Design review of the part built by this model. Coordinates are the model's own, in mm. A direction names the side the tool comes from. Coordinates: 2 decimals unless noted, no trailing zeros. Loops run counter-clockwise (first coordinate to the right, second up) from the corner with the lowest first, then second, coordinate; pieces in that order, holes last. Notation, with made-up numbers: (8, 70.5) -> (21, 70.5) arc R18 ccw to (21, 80.5) -> close; hole circle Ø10 at (31.25, 52). An arc over 180 degrees is marked (long way). Answer in a Markdown table with one row per item.
```python
from build123d import *

# Parameters (mm, degrees)
CHAMFER_1_SIZE      = 0.2
CHAMFER_2_SIZE      = 0.2
CUT_EXTRUDE_1_DEPTH = 2.4
EXTRUDE_2_REACH     = 21
SKETCH_4_R          = 1.832050808


with BuildPart() as part:
    # Sketch S → Revolve D (revolve)
    with BuildSketch(Plane(origin=(0, 0, 0), x_dir=(-1, 0, 0), z_dir=(0, 1, 0))):
        Polygon((0, 0), (2.75, 0), (2.75, -3), (1.5, -3), (1.5, -19), (0, -19), align=None)
    revolve(axis=Axis((0, 0, 20), (0, 0, -1)))

    # Chamfer 1
    chamfer_1_edges = [part.edges().sort_by_distance(p)[0] for p in [
        (2.75, 0, 0),
    ]]
    chamfer(chamfer_1_edges, length=CHAMFER_1_SIZE)

    # Chamfer 2
    chamfer_2_edges = [part.edges().sort_by_distance(p)[0] for p in [
        (1.5, 0, -19),
    ]]
    chamfer(chamfer_2_edges, length=CHAMFER_2_SIZE)

    # Sketch 2 → Cut-Extrude 1 (cut)
    with BuildSketch(Plane(origin=(0, 0, 0), x_dir=(0, 1, 0), z_dir=(0, 0, 1))):
        Polygon((0, 1.732050808), (1.5, 0.866025404), (1.5, -0.866025404), (0, -1.732050808), (-1.5, -0.866025404), (-1.5, 0.866025404), align=None)
    extrude(amount=-CUT_EXTRUDE_1_DEPTH, mode=Mode.SUBTRACT)

    # Sketch 3 → Cut-Revolve 1 (revolve, cut)
    with BuildSketch(Plane(origin=(0, 0, 0), x_dir=(1, 0, 0), z_dir=(0, 1, 0))):
        Polygon((-1.832050808, 0), (0, 0), (0, 3.4), (-1.832050808, 2.342264973), align=None)
    revolve(axis=Axis((0, 0, -30.07825812), (0, 0, 1)), mode=Mode.SUBTRACT)

    # Sketch 4 → Extrude 2 (add, up to next)
    with BuildSketch(Plane.XY, mode=Mode.PRIVATE) as extrude_2_sk1:
        Circle(SKETCH_4_R)
        Polygon((-1.732050808, 0), (-0.866025404, 1.5), (0.866025404, 1.5), (1.732050808, 0), (0.866025404, -1.5), (-0.866025404, -1.5), align=None, mode=Mode.SUBTRACT)
    extrude_2_tool1 = extrude(extrude_2_sk1.sketch, amount=-EXTRUDE_2_REACH, mode=Mode.PRIVATE) - part.part
    add(extrude_2_tool1.solids().sort_by_distance((-1.780233, 0, 0))[0])


solid = part.part
```
(1) Draft analysis for pull direction X (two halves, no side actions). For faces 4 (the conical face through (0.023, 0.106, -3.337)), 5 (the cylindrical face through (0.596, -2.685, -1.62)), 6 (the flat face through (0, -2, 0)), 7 (the flat face through (1.293, 0.761, -1.249)), state which applies: pulls with the +X half, pulls with the -X half, needs draft (parallel to the pull), parting line crosses it, or undercut.
Evaluation:
| item | result |
|---|---|
| face 4 | undercut |
| face 5 | parting line crosses it |
| face 6 | needs draft |
| face 7 | undercut |
(2) For pin 1 (3 mm diameter, centred on y = 2, z = -15, fed in from -X); pin 2 (1 mm diameter, centred on y = 0.5, z = -11.5, fed in from +X); pin 3 (3 mm diameter, centred on y = 2, z = -10, fed in from +X), all flat-tipped, find the tip position at first contact; note any pin that passes through.
Evaluation:
| item | result |
|---|---|
| pin 1 | stops at x = -1.41 |
| pin 2 | stops at x = 1.5 |
| pin 3 | stops at x = 1.41 |
(3) Tool access review of faces 1 (the flat face through (0, 0, -19)), 2 (the flat face through (0, -1.5, -1)), 3 (the cylindrical face through (1.5, 0.07, -11.01)): name each direction out of +Z, -Z, +X, -X, +Y, -Y from which nothing blocks a thin tool from reaching the whole face with its end or side.
Evaluation:
| item | result |
|---|---|
| face 1 | -Z, +X, -X, +Y, -Y |
| face 2 | +Z |
| face 3 | -Z |
(4) Take a section at A-A on z = -9.75. Give the boundary of the cut face in (x, y).
Evaluation:
| item | result |
|---|---|
| outline | circle Ø3 at (0, 0) |
(5) To check wall thickness, follow probe 1 along Z at (x, y) = (-2.1, 1.2); probe 2 along X at (y, z) = (-1.05, -1.75); probe 3 along X at (y, z) = (-0.05, -7). State the ranges of each line that lie inside material, in increasing order.
Evaluation:
| item | result |
|---|---|
| probe 1 | z = -3 to 0 |
| probe 2 | x = -2.54 to -1.13, 1.13 to 2.54 |
| probe 3 | x = -1.5 to 1.5 |
